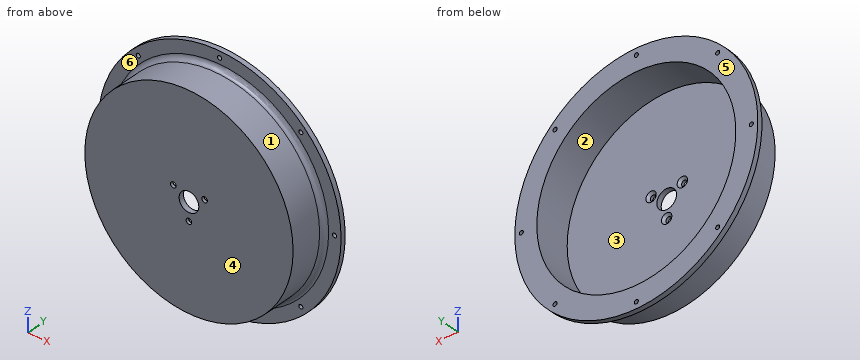
```python
from build123d import *

# Parameters (mm, degrees)
SKETCH1_R                                       = 63.5
SKETCH1_R_2                                     = 60.690000065
BOSS_EXTRUDE1_DEPTH                             = 25.4
SKETCH3_R                                       = 63.5
BOSS_EXTRUDE2_DEPTH                             = 3.175
CUT_EXTRUDE1_REACH                              = 27.4
SKETCH8_R                                       = 6
SKETCH9_R                                       = 74.095000033
SKETCH9_R_2                                     = 63.5
BOSS_EXTRUDE4_DEPTH                             = 3
M3X0_5_TAPPED_HOLE1_D                           = 2.5
CIRPATTERN2_COUNT                               = 8
FILLET1_R                                       = 3
CSK_FOR_M3_FLAT_HEAD_MACHINE_SCREW1_D           = 3.4
CSK_FOR_M3_FLAT_HEAD_MACHINE_SCREW1_CSINK_D     = 6.3
CSK_FOR_M3_FLAT_HEAD_MACHINE_SCREW1_CSINK_ANGLE = 90
CIRPATTERN3_COUNT                               = 3


with BuildPart() as part:
    # Sketch1 → Boss-Extrude1 (new body)
    with BuildSketch(Plane(origin=(0, 0, 0), x_dir=(1, 0, 0), z_dir=(0, 1, 0))):
        Circle(SKETCH1_R)
        Circle(SKETCH1_R_2, mode=Mode.SUBTRACT)
    extrude(amount=BOSS_EXTRUDE1_DEPTH)

    # Sketch3 → Boss-Extrude2 (add)
    with BuildSketch(Plane(origin=(0, 0, 0), x_dir=(1, 0, 0), z_dir=(0, 1, 0))):
        Circle(SKETCH3_R)
    extrude(amount=BOSS_EXTRUDE2_DEPTH)

    # Sketch8 → Cut-Extrude1 (cut, up to next)
    with BuildSketch(Plane.XZ, mode=Mode.PRIVATE) as cut_extrude1_sk1:
        Circle(SKETCH8_R)
    cut_extrude1_tool1 = extrude(cut_extrude1_sk1.sketch, amount=-CUT_EXTRUDE1_REACH, mode=Mode.PRIVATE) & part.part
    add(cut_extrude1_tool1.solids().sort_by_distance((0, 0, 0))[0], mode=Mode.SUBTRACT)

    # Sketch9 → Boss-Extrude4 (add)
    with BuildSketch(Plane(origin=(0, 25.4, 0), x_dir=(1, 0, 0), z_dir=(0, 1, 0))):
        Circle(SKETCH9_R)
        Circle(SKETCH9_R_2, mode=Mode.SUBTRACT)
    extrude(amount=-BOSS_EXTRUDE4_DEPTH)

    # M3x0.5 Tapped Hole1 (through all)
    with Locations(Plane(origin=(0, 25.4, 0), x_dir=(1, 0, 0), z_dir=(0, 1, 0))):
        with Locations((0, 70.1)):
            m3x0_5_tapped_hole1 = Hole(M3X0_5_TAPPED_HOLE1_D / 2)

    # CirPattern2: M3x0.5 Tapped Hole1 ×8 about axis
    cirpattern2_axis = Axis((0, 0, 0), (0, 1, 0))
    for i in range(1, CIRPATTERN2_COUNT):
        add(m3x0_5_tapped_hole1.rotate(cirpattern2_axis, i * 360 / CIRPATTERN2_COUNT), mode=Mode.SUBTRACT)

    # Fillet1
    fillet1_edges = [part.edges().sort_by_distance(p)[0] for p in [
        (-63.5, 22.4, 0),
    ]]
    fillet(fillet1_edges, radius=FILLET1_R)

    # CSK for M3 Flat Head Machine Screw1 (through all)
    with Locations(Plane(origin=(0, 3.175, 0), x_dir=(1, 0, 0), z_dir=(0, 1, 0))):
        with Locations((0, 11)):
            csk_for_m3_flat_head_machine_screw1 = CounterSinkHole(CSK_FOR_M3_FLAT_HEAD_MACHINE_SCREW1_D / 2, CSK_FOR_M3_FLAT_HEAD_MACHINE_SCREW1_CSINK_D / 2, counter_sink_angle=CSK_FOR_M3_FLAT_HEAD_MACHINE_SCREW1_CSINK_ANGLE)

    # CirPattern3: CSK for M3 Flat Head Machine Screw1 ×3 about axis
    cirpattern3_axis = Axis((0, 0, 0), (0, 1, 0))
    for i in range(1, CIRPATTERN3_COUNT):
        add(csk_for_m3_flat_head_machine_screw1.rotate(cirpattern3_axis, i * 360 / CIRPATTERN3_COUNT), mode=Mode.SUBTRACT)


solid = part.part
```
Geometry check sheet. Reference: the model listing, model coordinates, mm. Face numbers are marked on the shaded views. A direction names the side the tool comes from. Coordinates: 2 decimals unless noted, no trailing zeros. Order: outer loops, then holes, each group sorted by start corner. A loop starts at its lowest first (then second) coordinate and runs counter-clockwise, first axis right, second up.
Q1. Sectioned sample at A-A on y = 15.75. Record the cut outline in (x, z).
Reply:
outline: circle Ø127 at (0, 0); hole circle Ø121.38 at (0, 0)
Q2. Thickness scan on probe 1 along X at (y, z) = (23.05, 0) (3 decimals); probe 2 along X at (y, z) = (16.5, 0). Record the ranges inside material, lowest first.
Reply:
probe 1: x = -74.095 to -71.35, -68.85 to -60.69, 60.69 to 68.85, 71.35 to 74.095
probe 2: x = -63.5 to -60.69, 60.69 to 63.5
Q3. Depth check by flat-ended pin: pin 1 Ø5.5 at (x, z) = (9.53, 5.5) entering from +Y; pin 2 Ø12 at (y, z) = (8.5, -26) entering from +X; pin 3 Ø5 at (y, z) = (18.5, 9) entering from +X; pin 4 Ø3 at (x, z) = (-70.1, 0) entering from +Y. Enter the tip coordinate at first touch or a pass-through.
Reply:
pin 1: stops at y = 2.78
pin 2: stops at x = 60.27
pin 3: stops at x = 63.36
pin 4: stops at y = 25.4
Q4. Draft check along Z on the marked faces 1, 2, 3 and 4. Enter one of: released by +Z, released by -Z, zero draft, split by the parting line, or undercut.
Reply:
face 1: split by the parting line
face 2: undercut
face 3: undercut
face 4: zero draft
Q5. Tool access check on the marked faces 5 and 6. Record the directions out of +Z, -Z, +X, -X, +Y, -Y that give a thin tool (end or side, any length) a straight path to the whole face; none if there is none.
Reply:
face 5: +Z, -Z, +X, -X, +Y
face 6: -Y
